Part model, mm, in its own coordinate system. A direction names the side the tool comes from. Coordinates: 2 decimals unless noted, no trailing zeros. Loops run counter-clockwise (first coordinate to the right, second up) from the corner with the lowest first, then second, coordinate; pieces in that order, holes last. Notation, with made-up numbers: (-4.75, 27) -> (54.25, 27) arc R22 ccw to (54.25, 57) -> close; hole circle Ø1 at (5, 44.5). An arc over 180 degrees is marked (long way). Use one line per item in the form item = value. Start each with the question number.
(1) Band-saw the part on B-B on z = -0.5. Give the cut face in (x, y), then the cut area to 3 significant figures.
(2) 3-axis set-ups, long thin cutter, end or side, ignore diameter. For faces 4 (the flat face through (-2.4, 0.1, 4)), 5 (the cylindrical face through (-2.17, -9.76, 1.48)), 6 (the cylindrical face through (-1.23, -0.94, 3.53)): which of +Z, -Z, +X, -X, +Y, -Y reach the whole face in a straight line?
(3) Pin check, flat tips, straight feed: P1, Ø2, axis at x = 0, z = 0.25, coming from the +Y side; P2, Ø3, axis at x = -5.5, z = 0.5, coming from the -Y side; P3, Ø5, axis at y = -4, z = 9.5, coming from the +X side; P4, Ø3, axis at x = -7, z = 8, coming from the +Y side. Stop position of each tip, or through.
(4) Band-saw the part on A-A on y = 8.75. Give the cut face in (x, z), then the cut area to 3 significant figures.
(5) Drill centre lines: L1, parallel to Z at x = -8.75, y = -5.25; L2, parallel to X at y = -3, z = 3.25; L3, parallel to X at y = -7, z = 5.75. Where is each one in solid material? Low to high. Write a range as [from, to].
(6) Mould opens along Y. For faces 1 (the cylindrical face through (10, 3.2, 7.9)), 2 (the flat face through (5, -9, 16)), 3 (the cylindrical face through (-6.945, 5.989, 3.493)) say: +Y half, -Y half, draft (parallel to the pull), parting line (faces both ways), or undercut.
(7) Band-saw the part on D-D on z = 7. Give the cut face in (x, y).
(8) Band-saw the part on C-C on y = 5.75. Give the cut face in (x, z), then the cut area to 3 significant figures.
```python
from build123d import *

# Parameters (mm, degrees)
CYLINDER039_R          = 2.25
CYLINDER039_DEPTH      = 30
ARRAY002_COUNT         = 8
CYLINDER038_R          = 1.55
CYLINDER038_DEPTH      = 30
CYLINDER045_R          = 1.25
CYLINDER045_DEPTH      = 32
CYLINDER045_ROLL_ANGLE = 90
CYLINDER043_R          = 3.5
CYLINDER043_DEPTH      = 5.5
CYLINDER042_R          = 10
CYLINDER042_DEPTH      = 16
CYLINDER037_R          = 10
CYLINDER037_DEPTH      = 16
CYLINDER036_R          = 10.5
CYLINDER036_DEPTH      = 16
CYLINDER044_R          = 2
CYLINDER044_DEPTH      = 5.5
CHAMFER062_1_SIZE      = 0.3
CHAMFER062_2_SIZE      = 0.2
CHAMFER062_3_SIZE      = 0.1


with BuildPart() as array002:
    # Cylinder039 → Cylinder039 (new body)
    with BuildSketch(Plane(origin=(7, 0, -10), x_dir=(1, 0, 0), z_dir=(0, 0, 1))):
        Circle(CYLINDER039_R)
    extrude(amount=CYLINDER039_DEPTH)

    # Array002: Array002 ×8 about axis
    array002_axis = Axis((0, 0, 0), (0, 0, 1))


with BuildPart() as array002_1:
    add(array002.part)
    for i in range(1, ARRAY002_COUNT):
        add(array002.part.rotate(array002_axis, i * 360 / ARRAY002_COUNT))


with BuildPart() as fusion033:
    # Cylinder038 → Cylinder038 (new body)
    with BuildSketch(Plane.XY.offset(-10)):
        Circle(CYLINDER038_R)
    extrude(amount=CYLINDER038_DEPTH)

    # Fusion033: union Array002
    add(array002_1.part)


with BuildPart() as cylinder045:
    # Cylinder045 → Cylinder045 (new body)
    with BuildSketch(Plane.XY):
        Circle(CYLINDER045_R)
    extrude(amount=CYLINDER045_DEPTH)


with BuildPart() as cylinder045_1:
    # Cylinder045 roll: moved
    add(cylinder045.part.rotate(Axis((0, 0, 0), (1, 0, 0)), CYLINDER045_ROLL_ANGLE))


with BuildPart() as cylinder045_2:
    # Cylinder045 placement: moved
    add(cylinder045_1.part.moved(Location((0, 15, 0.25))))


with BuildPart() as cylinder043:
    # Cylinder043 → Cylinder043 (new body)
    with BuildSketch(Plane.XY.offset(-2)):
        Circle(CYLINDER043_R)
    extrude(amount=CYLINDER043_DEPTH)


with BuildPart() as cylinder042:
    # Cylinder042 → Cylinder042 (new body)
    with BuildSketch(Plane.XY.offset(-13)):
        Circle(CYLINDER042_R)
    extrude(amount=CYLINDER042_DEPTH)


with BuildPart() as fusion034:
    # Cylinder037 → Cylinder037 (new body)
    with BuildSketch(Plane.XY.offset(4)):
        Circle(CYLINDER037_R)
    extrude(amount=CYLINDER037_DEPTH)

    # Fusion034: union Cylinder042
    add(cylinder042.part)


with BuildPart() as cut028:
    # Cylinder036 → Cylinder036 (new body)
    with BuildSketch(Plane.XY):
        Circle(CYLINDER036_R)
    extrude(amount=CYLINDER036_DEPTH)

    # Cut028: cut Fusion034
    add(fusion034.part, mode=Mode.SUBTRACT)


with BuildPart() as chamfer062:
    # Cylinder044 → Cylinder044 (new body)
    with BuildSketch(Plane.XY.offset(3.5)):
        Circle(CYLINDER044_R)
    extrude(amount=CYLINDER044_DEPTH)

    # Fusion035: union Cylinder043, Cut028
    add(cylinder043.part)
    add(cut028.part)

    # Cut002: cut Cylinder045
    add(cylinder045_2.part, mode=Mode.SUBTRACT)

    # Cut029: cut Fusion033
    add(fusion033.part, mode=Mode.SUBTRACT)

    # Chamfer062 1
    chamfer062_1_edges = [chamfer062.edges().sort_by_distance(p)[0] for p in [
        (-1.55, 0, -2),
    ]]
    chamfer(chamfer062_1_edges, length=CHAMFER062_1_SIZE)

    # Chamfer062 2
    chamfer062_2_edges = [chamfer062.edges().sort_by_distance(p)[0] for p in [
        (-3.5, 0, -2),
    ]]
    chamfer(chamfer062_2_edges, length=CHAMFER062_2_SIZE)

    # Chamfer062 3
    chamfer062_3_edges = [chamfer062.edges().sort_by_distance(p)[0] for p in [
        (-1.55, 0, 9),
    ]]
    chamfer(chamfer062_3_edges, length=CHAMFER062_3_SIZE)


solid = chamfer062.part
```
A:
q1.outline = (-1, -3.35) -> (-1, -1.18) arc R1.55 cw to (-1, 1.18) -> (-1, 3.35) arc R3.5 ccw to start; (1, -3.35) arc R3.5 ccw to (1, 3.35) -> (1, 1.18) arc R1.55 cw to (1, -1.18) -> close
q1.area = 22.9 mm²
q2.face_4 = +Z
q2.face_5 = -Z
q2.face_6 = +Z, -Z
q3.P1 = through
q3.P2 = -9.71
q3.P3 = 10.39
q3.P4 = 8.94
q4.outline = (-5.8, 0) -> (-4.84, 0) -> (-4.84, 3) -> (-1.41, 3) -> (-1.41, 4) -> (-4.84, 4) -> (-4.84, 16) -> (-5.8, 16) -> close; (1.41, 3) -> (4.84, 3) -> (4.84, 0) -> (5.8, 0) -> (5.8, 16) -> (4.84, 16) -> (4.84, 4) -> (1.41, 4) -> close
q4.area = 37.7 mm²
q5.L1 = [0, 16]
q5.L2 = [-10.06, -6.07], [-3.83, 3.83], [6.07, 10.06]
q5.L3 = [-7.83, -7.14], [7.14, 7.83]
q6.face_1 = parting line
q6.face_2 = draft
q6.face_3 = undercut
q7.outline = circle Ø21 at (0, 0); circle Ø4 at (0, 0); hole circle Ø20 at (0, 0); hole circle Ø3.1 at (0, 0)
q8.outline = (-8.79, 0) -> (-8.18, 0) -> (-8.18, 3) -> (-7.05, 3) -> (-7.05, 4) -> (-8.18, 4) -> (-8.18, 16) -> (-8.79, 16) -> close; (-2.85, 3) -> (-1.87, 3) -> (-1.87, 4) -> (-2.85, 4) -> close; (1.87, 3) -> (2.85, 3) -> (2.85, 4) -> (1.87, 4) -> close; (7.05, 3) -> (8.18, 3) -> (8.18, 0) -> (8.79, 0) -> (8.79, 16) -> (8.18, 16) -> (8.18, 4) -> (7.05, 4) -> close
q8.area = 23.5 mm²
